Part model, mm, in its own coordinate system. Face numbers are marked on the shaded views. A direction names the side the tool comes from. Coordinates: 2 decimals unless noted, no trailing zeros. Write each loop counter-clockwise with the first axis right and the second up, starting at its lowest first coordinate (ties: lowest second). Pieces come first, ordered by that corner, then holes. Notation, with made-up numbers: (61.25, 28) - (67.25, 28) arc R34 cw to (67.25, 59) - close; hole circle Ø11 at (-16.75, -12). An arc over 180 degrees is marked (long way). Write each question's results on one line, items separated by ' | '.
from build123d import *

# Parameters (mm, degrees)
F0_W     = 42
F0_H     = 14.25
F0_W_2   = 38
F0_H_2   = 10.25
F1_DEPTH = 1
F2_DEPTH = 20
F4_D     = 5.5
F4_DEPTH = 14.4


with BuildPart() as f1:
    # F0 (on Top) → F1 (new body)
    with BuildSketch(Plane.XY):
        Rectangle(F0_W, F0_H)
        Rectangle(F0_W_2, F0_H_2, mode=Mode.SUBTRACT)
        Rectangle(F0_W_2, F0_H_2)
    extrude(amount=F1_DEPTH)

    # F0 (on Top) → F2 (join)
    with BuildSketch(Plane.XY):
        Rectangle(F0_W, F0_H)
        Rectangle(F0_W_2, F0_H_2, mode=Mode.SUBTRACT)
    extrude(amount=-F2_DEPTH)

    # F4
    with Locations(Plane.YZ.offset(21)):
        with Locations((0, -10)):
            Hole(F4_D / 2, depth=F4_DEPTH)


solid = f1.part
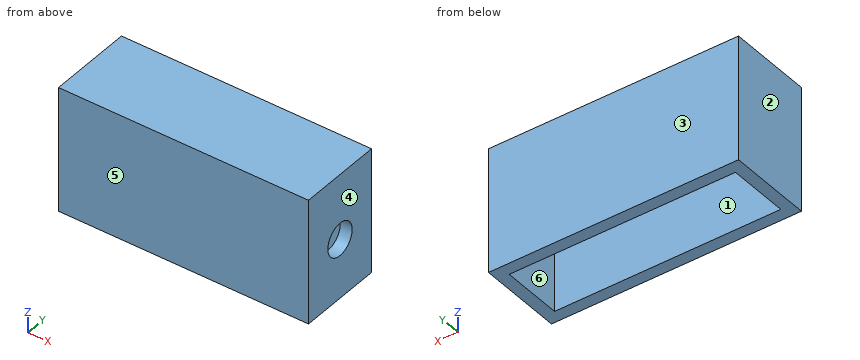
(1) Two-plate mould, pull along X, no slides. Class the marked faces 1, 2, 3 and 4: released by +X, released by -X, zero draft, split by the parting line, or undercut.
Return value:
face 1: undercut | face 2: released by -X | face 3: zero draft | face 4: released by +X
(2) 3-axis set-ups, long thin cutter, end or side, ignore diameter. For the marked faces 5 and 6: which of +Z, -Z, +X, -X, +Y, -Y reach the whole face in a straight line?
Return value:
face 5: +Z, -Z, +X, -X, -Y | face 6: -Z
(3) Saw through at A-A on y = 0. Write the cut outline in (x, z).
Return value:
outline: (-21, -20) - (-19, -20) - (-19, 0) - (19, 0) - (19, -7.25) - (21, -7.25) - (21, 1) - (-21, 1) - close; (19, -20) - (21, -20) - (21, -12.75) - (19, -12.75) - close
(4) Saw through at C-C on x = 4. Write the cut outline in (y, z) (3 decimals).
Return value:
outline: (-7.125, -20) - (-5.125, -20) - (-5.125, 0) - (5.125, 0) - (5.125, -20) - (7.125, -20) - (7.125, 1) - (-7.125, 1) - close
(5) Saw through at B-B on z = -5.25. Write the cut outline in (x, y) (3 decimals).
Return value:
outline: (-21, -7.125) - (21, -7.125) - (21, 7.125) - (-21, 7.125) - close; hole (-19, -5.125) - (19, -5.125) - (19, 5.125) - (-19, 5.125) - close
(6) Saw through at D-D on z = -10. Write the cut outline in (x, y) (3 decimals).
Return value:
outline: (-21, -7.125) - (21, -7.125) - (21, -2.75) - (19, -2.75) - (19, -5.125) - (-19, -5.125) - (-19, 5.125) - (19, 5.125) - (19, 2.75) - (21, 2.75) - (21, 7.125) - (-21, 7.125) - close
(7) Flat gauge pins, fed straight in: P1, Ø3, axis at y = -0.5, z = -11, coming from the +X side; P2, Ø6, axis at x = 0, y = 1, coming from the -Z side. Where does each tip first touch, or does it go through?
Return value:
P1: stops at x = -19 | P2: stops at z = 0
(8) Wall check: line 1 (X direction, y = -4.75, z = -17.75); line 2 (Y direction, x = -11, z = -1.25) (3 decimals); line 3 (Z direction, x = 19.5, y = 0). Give the ranges that are in metal, low to high. Write a range as from..to.
Return value:
line 1: x = -21..-19, 19..21 | line 2: y = -7.125..-5.125, 5.125..7.125 | line 3: z = -20..-12.75, -7.25..1
